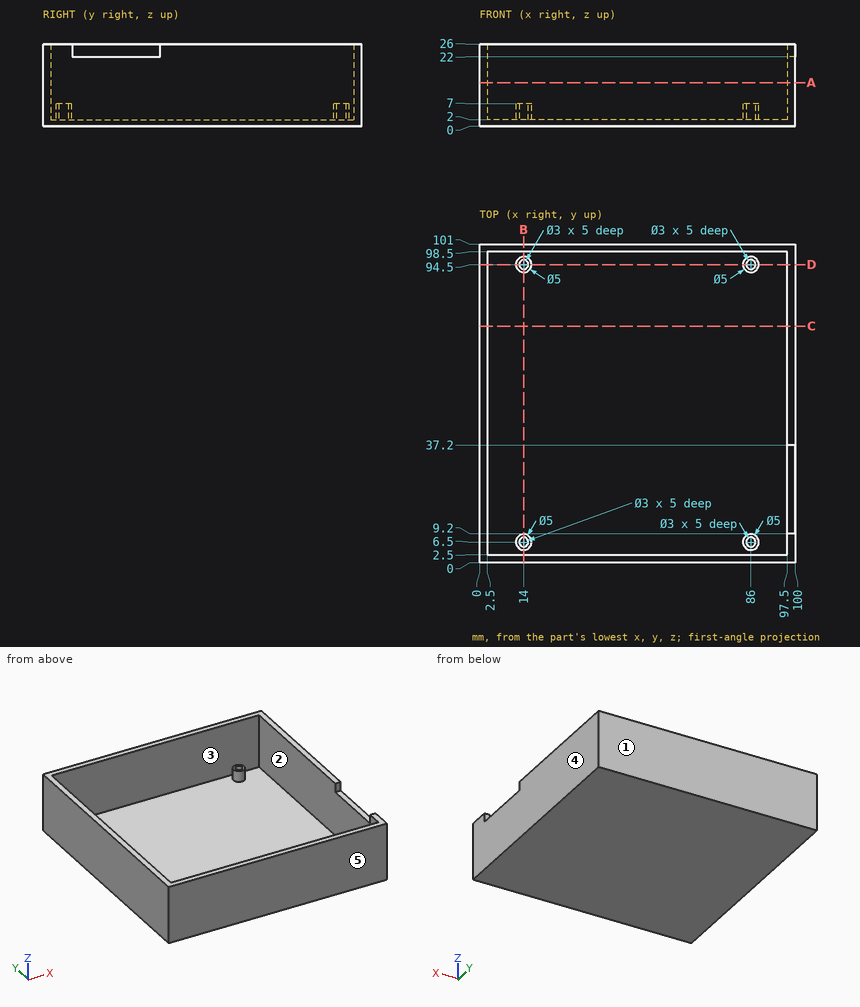
Answer from the drawing. Dimensions are ordinates in mm from the lowest x, y and z of the part. A direction names the side the tool comes from. Round coordinates to 2 decimals unless told otherwise and drop trailing zeros. Write each loop counter-clockwise with the first axis right and the second up, starting at its lowest first coordinate (ties: lowest second). Pieces come first, ordered by that corner, then holes. Notation, with made-up numbers: (28.5, 11.25) -> (59.5, 11.25) arc R12 ccw to (59.5, 15.25) -> close; hole circle Ø5 at (-33, 12). An arc over 180 degrees is marked (long way). Answer in a Markdown table with one row per item. Add a question column.
1) Which of the six approach directions +Z, -Z, +X, -X, +Y, -Y give full straight-line access (tool end or side, diameter ignored) to the marked faces 1 and 2?
2) Consider line 1 (Y direction, x = 86, z = 5.75); line 2 (X direction, y = 7.5, z = 19); line 3 (Y direction, x = 55, z = 5.25). Determine where each line is inside the solid, lowest interval first.
3) Find section B-B, the plane x = 14. Determine the outline of the cut face in (y, z), and give its area (3 significant figures).
4) Find section C-C, the plane y = 75. Determine the outline of the cut face in (x, z).
5) Determine the mould class of the marked faces 3, 4 and 5 for opening direction X: pulls with the +X half, pulls with the -X half, needs draft (parallel to the pull), parting line crosses it, or undercut.
6) Find section D-D, the plane y = 94.5. Determine the outline of the cut face in (x, z).
7) Find section A-A, the plane z = 13.75. Determine the outline of the cut face in (x, y), and give its area (3 significant figures).
8) Given P1, Ø4, axis at x = 15, y = 95, coming from the +Z side; P2, Ø2.5, axis at x = 86, y = 94.5, coming from the +Z side; P3, Ø1.2, axis at x = 99, y = 28, coming from the +Z side, each flat-ended and moving along its own axis, determine where each tip first touches the part or whether it passes through.
Findings below:
| question | item | result |
|---|---|---|
| 1 | face 1 | +Z, -Z, +X, -X, +Y |
| 1 | face 2 | +Z |
| 2 | line 1 | 0 to 2.5, 4 to 5, 8 to 9, 92 to 93, 96 to 97, 98.5 to 101 |
| 2 | line 2 | 0 to 2.5, 97.5 to 100 |
| 2 | line 3 | 0 to 2.5, 98.5 to 101 |
| 3 | outline | (0, 0) -> (101, 0) -> (101, 26) -> (98.5, 26) -> (98.5, 2) -> (97, 2) -> (97, 7) -> (96, 7) -> (96, 2) -> (93, 2) -> (93, 7) -> (92, 7) -> (92, 2) -> (9, 2) -> (9, 7) -> (8, 7) -> (8, 2) -> (5, 2) -> (5, 7) -> (4, 7) -> (4, 2) -> (2.5, 2) -> (2.5, 26) -> (0, 26) -> close |
| 3 | area | 342 mm² |
| 4 | outline | (0, 0) -> (100, 0) -> (100, 26) -> (97.5, 26) -> (97.5, 2) -> (2.5, 2) -> (2.5, 26) -> (0, 26) -> close |
| 5 | face 3 | undercut |
| 5 | face 4 | pulls with the +X half |
| 5 | face 5 | needs draft |
| 6 | outline | (0, 0) -> (100, 0) -> (100, 26) -> (97.5, 26) -> (97.5, 2) -> (88.5, 2) -> (88.5, 7) -> (87.5, 7) -> (87.5, 2) -> (84.5, 2) -> (84.5, 7) -> (83.5, 7) -> (83.5, 2) -> (16.5, 2) -> (16.5, 7) -> (15.5, 7) -> (15.5, 2) -> (12.5, 2) -> (12.5, 7) -> (11.5, 7) -> (11.5, 2) -> (2.5, 2) -> (2.5, 26) -> (0, 26) -> close |
| 7 | outline | (0, 0) -> (100, 0) -> (100, 101) -> (0, 101) -> close; hole (2.5, 2.5) -> (97.5, 2.5) -> (97.5, 98.5) -> (2.5, 98.5) -> close |
| 7 | area | 980 mm² |
| 8 | P1 | z = 7 |
| 8 | P2 | z = 2 |
| 8 | P3 | z = 22 |
